```python
from build123d import *

# Parameters (mm, degrees)
SKETCH1_W           = 56.5
SKETCH1_H           = 56.5
SKETCH1_W_2         = 50.5
SKETCH1_H_2         = 50.5
SKETCH1_R           = 1.65
BOSS_EXTRUDE1_DEPTH = 8.6
SKETCH2_W           = 50.5
SKETCH2_H           = 50.5
SKETCH2_W_2         = 44.5
SKETCH2_H_2         = 44.5
BOSS_EXTRUDE2_DEPTH = 2
BOSS_EXTRUDE3_START = 6.6
SKETCH4_W           = 50.5
SKETCH4_H           = 50.5
SKETCH4_W_2         = 44.5
SKETCH4_H_2         = 44.5
BOSS_EXTRUDE3_DEPTH = 2
CUT_EXTRUDE1_START  = 2
SKETCH5_W           = 6
SKETCH5_H           = 17.961455198
CUT_EXTRUDE1_DEPTH  = 4.6
SKETCH6_W           = 87.3205389
SKETCH6_H           = 82.15723747
CUT_EXTRUDE2_DEPTH  = 2.3
CUT_EXTRUDE4_DEPTH  = 10
SKETCH8_W           = 8
SKETCH8_H           = 40.5
BOSS_EXTRUDE4_DEPTH = 6.3


with BuildPart() as part:
    # Sketch1 → Boss-Extrude1 (new body)
    with BuildSketch(Plane(origin=(0, 0, 0), x_dir=(1, 0, 0), z_dir=(0, 1, 0))):
        Rectangle(SKETCH1_W, SKETCH1_H)
        Rectangle(SKETCH1_W_2, SKETCH1_H_2, mode=Mode.SUBTRACT)
        Polygon((-28.25, -28.25), (-28.25, -12.25), (-36.25, -20.25), (-36.25, -30.25), (-32.25, -34.25), (-24.25, -34.25), (-18.25, -28.25), align=None)
        with Locations((-32.25, -24.25)):
            Circle(SKETCH1_R, mode=Mode.SUBTRACT)
        Polygon((28.25, -28.25), (18.25, -28.25), (24.25, -34.25), (32.25, -34.25), (36.25, -30.25), (36.25, -20.25), (28.25, -12.25), align=None)
        with Locations((32.25, -24.25)):
            Circle(SKETCH1_R, mode=Mode.SUBTRACT)
        Polygon((24.25, 34.25), (18.25, 28.25), (28.25, 28.25), (28.25, 12.25), (36.25, 20.25), (36.25, 30.25), (32.25, 34.25), align=None)
        with Locations((32.25, 24.25)):
            Circle(SKETCH1_R, mode=Mode.SUBTRACT)
        Polygon((-36.25, 20.25), (-28.25, 12.25), (-28.25, 28.25), (-18.25, 28.25), (-24.25, 34.25), (-32.25, 34.25), (-36.25, 30.25), align=None)
        with Locations((-32.25, 24.25)):
            Circle(SKETCH1_R, mode=Mode.SUBTRACT)
    extrude(amount=BOSS_EXTRUDE1_DEPTH)

    # Sketch2 → Boss-Extrude2 (add)
    with BuildSketch(Plane(origin=(0, 0, 0), x_dir=(1, 0, 0), z_dir=(0, 1, 0))):
        Rectangle(SKETCH2_W, SKETCH2_H)
        Rectangle(SKETCH2_W_2, SKETCH2_H_2, mode=Mode.SUBTRACT)
    extrude(amount=BOSS_EXTRUDE2_DEPTH)

    # Sketch4 → Boss-Extrude3 (add)
    with BuildSketch(Plane(origin=(0, 0, 0), x_dir=(1, 0, 0), z_dir=(0, 1, 0)).offset(BOSS_EXTRUDE3_START)):
        Rectangle(SKETCH4_W, SKETCH4_H)
        Rectangle(SKETCH4_W_2, SKETCH4_H_2, mode=Mode.SUBTRACT)
    extrude(amount=BOSS_EXTRUDE3_DEPTH)

    # Sketch5 → Cut-Extrude1 (cut)
    with BuildSketch(Plane(origin=(0, 0, 0), x_dir=(1, 0, 0), z_dir=(0, 1, 0)).offset(CUT_EXTRUDE1_START)):
        with Locations((-22.25, 28.869783692)):
            Rectangle(SKETCH5_W, SKETCH5_H)
        with Locations((22.25, 28.869783692)):
            Rectangle(SKETCH5_W, SKETCH5_H)
    extrude(amount=CUT_EXTRUDE1_DEPTH, mode=Mode.SUBTRACT)

    # Sketch6 → Cut-Extrude2 (cut)
    with BuildSketch(Plane.XZ):
        with Locations((1.898272585, -1.518618068)):
            Rectangle(SKETCH6_W, SKETCH6_H)
    extrude(amount=-CUT_EXTRUDE2_DEPTH, mode=Mode.SUBTRACT)

    # Sketch7 → Cut-Extrude4 (cut)
    with BuildSketch(Plane(origin=(0, 8.6, 0), x_dir=(1, 0, 0), z_dir=(0, 1, 0))):
        Polygon((-36.25, -30.25), (-36.25, -28.25), (-40.881768663, -28.25), (-40.881768663, -34.995320637), (0, -34.995320637), (0, -28.25), (-18.25, -28.25), (-24.25, -34.25), (-32.25, -34.25), align=None)
        Polygon((18.25, -28.25), (0, -28.25), (0, -34.995320637), (39.184342226, -34.995320637), (39.184342226, -28.25), (36.25, -28.25), (36.25, -30.25), (32.25, -34.25), (24.25, -34.25), align=None)
        Polygon((36.25, 20.25), (36.25, -20.25), (28.25, -12.25), (28.25, 12.25), align=None)
        Polygon((-36.25, 20.25), (-36.25, -20.25), (-28.25, -12.25), (-28.25, 12.25), align=None)
        Polygon((-36.25, 30.25), (-36.25, 28.25), (-18.25, 28.25), (-24.25, 34.25), (-32.25, 34.25), align=None)
        Polygon((-38.207606214, 28.25), (-36.25, 28.25), (-36.25, 30.25), (-32.25, 34.25), (-24.25, 34.25), (-18.25, 28.25), (0, 28.25), (0, 36.724555445), (-38.207606214, 36.724555445), align=None)
        Polygon((28.25, 12.25), (36.25, 20.25), (28.25, 20.25), align=None)
        Polygon((28.25, -20.25), (36.25, -20.25), (28.25, -12.25), align=None)
        Polygon((-18.25, -28.25), (-36.25, -28.25), (-36.25, -30.25), (-32.25, -34.25), (-24.25, -34.25), align=None)
        Polygon((-28.25, -12.25), (-36.25, -20.25), (-28.25, -20.25), align=None)
        Polygon((-28.25, 20.25), (-36.25, 20.25), (-28.25, 12.25), align=None)
        Polygon((24.25, 34.25), (18.25, 28.25), (36.25, 28.25), (36.25, 30.25), (32.25, 34.25), align=None)
        Polygon((0, 36.724555445), (0, 28.25), (18.25, 28.25), (24.25, 34.25), (32.25, 34.25), (36.25, 30.25), (36.25, 28.25), (40.981198071, 28.25), (40.981198071, 36.724555445), align=None)
        Polygon((36.25, -28.25), (18.25, -28.25), (24.25, -34.25), (32.25, -34.25), (36.25, -30.25), align=None)
    extrude(amount=-CUT_EXTRUDE4_DEPTH, mode=Mode.SUBTRACT)

    # Sketch8 → Boss-Extrude4 (add)
    with BuildSketch(Plane(origin=(0, 8.6, 0), x_dir=(1, 0, 0), z_dir=(0, 1, 0))):
        with Locations((-32.25, 0)):
            Rectangle(SKETCH8_W, SKETCH8_H)
        with Locations((32.25, 0)):
            Rectangle(SKETCH8_W, SKETCH8_H)
    extrude(amount=-BOSS_EXTRUDE4_DEPTH)


solid = part.part
```
Model file for the job. Use its own axes, mm. A direction names the side the tool comes from. Coordinates: 2 decimals unless noted, no trailing zeros. Order: outer loops, then holes, each group sorted by start corner. A loop starts at its lowest first (then second) coordinate and runs counter-clockwise, first axis right, second up. Notation, with made-up numbers: (72, -37) - (99, -37) arc R12 ccw to (99, -22) - close; hole circle Ø7 at (-37, 5.5). An arc over 180 degrees is marked (long way). Return JSON: item names as keys, results as strings. Group by question number.
1) Saw through at A-A, the plane y = 4.5. Write the cut outline in (x, z).
2) Mould opens along Z. For faces 1 (the flat face through (-1, 5, -28.25)), 2 (the flat face through (0, 6.6, -23)), 3 (the flat face through (0, 2.3, -27)) say: released by +Z, released by -Z, zero draft, split by the parting line, or undercut.
3) Tool access for faces 4 (the flat face through (0, 4, 25.25)), 5 (the flat face through (-25.25, 4, -1)), 6 (the flat face through (0, 8, 22.25)): list every direction of +Z, -Z, +X, -X, +Y, -Y with a clear straight run to the whole face (end or side of a thin tool).
4) Probe line 1 (Z direction, x = -32.25, y = 3.75); line 2 (X direction, y = 4, z = -24.25); line 3 (X direction, y = 7.25, z = -24.25). List the from-to ranges inside material, lowest first. Write a range as from..to.
5) Saw through at B-B, the plane z = -24.25. Write the cut outline in (x, y).
6) Saw through at C-C, the plane x = -4.5. Write the cut outline in (y, z), plus the area to 3 significant figures.
7) Flat gauge pin, fed straight in: P1, Ø25, axis at x = -10, z = -11, coming from the -Y side. Where does the tip first touch, or does it go through?
8) Saw through at D-D, the plane z = -11.5. Write the cut outline in (x, y).
Values found:
{
 "1": {"outline": "(-36.25, -28.25) - (-25.25, -28.25) - (-25.25, 25.25) - (25.25, 25.25) - (25.25, -28.25) - (36.25, -28.25) - (36.25, 28.25) - (-36.25, 28.25) - close; (-19.25, -28.25) - (19.25, -28.25) - (19.25, -25.25) - (-19.25, -25.25) - close; hole circle Ø3.3 at (-32.25, -24.25); hole circle Ø3.3 at (-32.25, 24.25); hole circle Ø3.3 at (32.25, -24.25); hole circle Ø3.3 at (32.25, 24.25)"},
 "2": {"face 1": "released by -Z", "face 2": "undercut", "face 3": "zero draft"},
 "3": {"face 4": "-Y", "face 5": "-Z, -Y", "face 6": "+Y, -Y"},
 "4": {"line 1": "z = -28.25..-25.9, -22.6..22.6, 25.9..28.25", "line 2": "x = -36.25..-33.9, -30.6..-25.25, 25.25..30.6, 33.9..36.25", "line 3": "x = -36.25..-33.9, -30.6..30.6, 33.9..36.25"},
 "5": {"outline": "(-36.25, 2.3) - (-33.9, 2.3) - (-33.9, 8.6) - (-36.25, 8.6) - close; (-30.6, 2.3) - (-25.25, 2.3) - (-25.25, 6.6) - (25.25, 6.6) - (25.25, 2.3) - (30.6, 2.3) - (30.6, 8.6) - (-30.6, 8.6) - close; (33.9, 2.3) - (36.25, 2.3) - (36.25, 8.6) - (33.9, 8.6) - close"},
 "6": {"outline": "(2.3, -28.25) - (8.6, -28.25) - (8.6, -22.25) - (6.6, -22.25) - (6.6, -25.25) - (2.3, -25.25) - close; (2.3, 25.25) - (6.6, 25.25) - (6.6, 22.25) - (8.6, 22.25) - (8.6, 28.25) - (2.3, 28.25) - close", "area": "49.8 mm²"},
 "7": {"P1": "stops at y = 6.6"},
 "8": {"outline": "(-36.25, 2.3) - (-25.25, 2.3) - (-25.25, 6.6) - (-22.25, 6.6) - (-22.25, 8.6) - (-36.25, 8.6) - close; (22.25, 6.6) - (25.25, 6.6) - (25.25, 2.3) - (36.25, 2.3) - (36.25, 8.6) - (22.25, 8.6) - close"}
}
